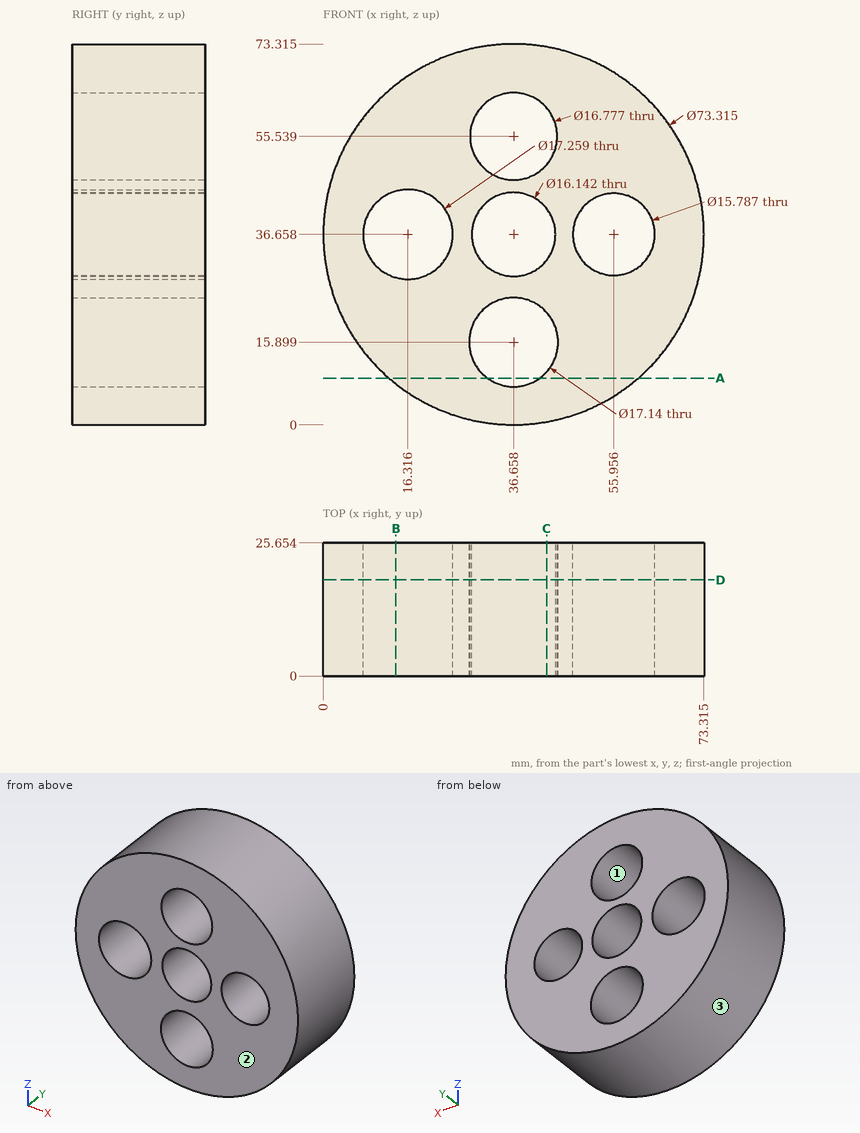
Geometry: see drawing. Coordinates: mm, zero at the bounding-box minimum. Round coordinates to 2 decimals unless told otherwise and drop trailing zeros. Write each loop counter-clockwise with the first axis right and the second up, starting at its lowest first coordinate (ties: lowest second). Pieces come first, ordered by that corner, then holes. Notation, with made-up numbers: M -8,15 L 17,15 A18 ccw 17,40 Z; hole C 35,7 d6. An arc over 180 degrees is marked long. Answer as a JSON object with one key per item and string values. Group by question number.
(1) Section query C-C on x = 43. Output: boundary loops of the cut face in (y, z) (1 decimal), then the cut area to 3 significant figures.
(2) Ray query, line 1 (Z direction, x = 40, y = 16) (1 decimal); line 2 (Z direction, x = 34.5, y = 10) (1 decimal); line 3 (X direction, y = 21.75, z = 39) (1 decimal). Return the intervals inside material, ascending. Write a range as [from, to].
(3) Section query A-A on z = 9. Output: boundary loops of the cut face in (x, y).
(4) Mould query, pull axis Z, two halves, no side actions, for the marked faces 1, 2 and 3. Classes: +Z half, -Z half, draft (parallel to the pull), parting line (faces both ways), or undercut.
(5) First-contact query: pin 1 (8 mm diameter, centred on x = 25, y = 9, fed in from -Z); pin 2 (5 mm diameter, centred on y = 11, z = 13.5, fed in from +X); pin 3 (4 mm diameter, centred on y = 15.5, z = 8, fed in from +X); pin 4 (10 mm diameter, centred on x = 36.66, z = 55.54, fed in from +Y). Flat tips, straight axial feed; report the tip coordinate or a pass-through.
(6) Section query B-B on x = 14. Output: boundary loops of the cut face in (y, z) (1 decimal), then the cut area to 3 significant figures.
(7) Section query D-D on y = 18.5. State how many separate pieces and enclosed holes the cut face has, then the cut area to 3 significant figures.
Computed values:
{
 "1": {"outline": "M 0,0.6 L 25.7,0.6 L 25.7,10.1 L 0,10.1 Z; M 0,21.7 L 25.7,21.7 L 25.7,31.7 L 0,31.7 Z; M 0,41.6 L 25.7,41.6 L 25.7,50 L 0,50 Z; M 0,61 L 25.7,61 L 25.7,72.8 L 0,72.8 Z", "area": "1,020 mm^2"},
 "2": {"line 1": "[0.2, 8], [23.8, 29.3], [44, 47.8], [63.2, 73.2]", "line 2": "[0.1, 7.6], [24.2, 28.9], [44.4, 47.4], [63.6, 73.3]", "line 3": "[0.1, 8], [24.6, 28.9], [44.4, 48.4], [63.5, 73.2]"},
 "3": {"outline": "M 12.6,0 L 31.57,0 L 31.57,25.65 L 12.6,25.65 Z; M 41.74,0 L 60.72,0 L 60.72,25.65 L 41.74,25.65 Z"},
 "4": {"face 1": "undercut", "face 2": "draft", "face 3": "parting line"},
 "5": {"pin 1": "z = 0.81", "pin 2": "x = 66.94", "pin 3": "x = 61.82", "pin 4": "through"},
 "6": {"outline": "M 0,7.8 L 25.7,7.8 L 25.7,28.3 L 0,28.3 Z; M 0,45 L 25.7,45 L 25.7,65.5 L 0,65.5 Z", "area": "1,050 mm^2"},
 "7": {"separate pieces": "1", "enclosed holes": "5", "area": "3,140 mm^2"}
}
